Autodesk Inventor part; units mm, degrees
ref_plane "YZ Plane" through (0, 0, 0) normal (1, 0, 0) x (0, 1, 0)
ref_plane "XZ Plane" through (0, 0, 0) normal (0, 1, 0) x (-1, 0, 0)
ref_plane "XY Plane" through (0, 0, 0) normal (0, 0, 1) x (1, 0, 0)
sketch "Schizzo3" plane through (0, 0, 0) normal (0, 0, 1) x (1, 0, 0)
  line L0 (-46, 0) -> (-46, 3)
  line L1 (-46, 3) -> (46, 3)
  line L2 (46, 3) -> (46, 0)
  line L3 (46, 0) -> (61, 0)
  line L4 (61, 0) -> (61, 18)
  line L5 (61, 18) -> (-61, 18)
  line L6 (-61, 18) -> (-61, 0)
  line L7 (-61, 0) -> (-46, 0)
  line L8 (0, 0) -> (0, 18)
  point P0 (0, 3)
  dimension "d10" = 122
  dimension "d11" = 92
  dimension "d12" = 18
  dimension "d13" = 3
extrude "Estrusione1" add sketch "Schizzo3" along normal mid plane 90
sketch "Schizzo4" plane through (-61, 18, 45) normal (0, 1, 0) x (1, 0, 0)
  line L0 (0, 90) -> (0, 0)
  line L1 (0, 90) -> (122, 90)
  line L2 (17, 60) -> (35, 60)
  line L3 (35, 60) -> (35, 30)
  line L4 (35, 30) -> (17, 30)
  line L5 (17, 30) -> (17, 60)
  line L6 (0, 45) -> (122, 45) construction
  line L7 (122, 90) -> (122, 0) construction
  circle A0 centre (17, 60) radius 1.5
  circle A1 centre (35, 60) radius 1.5
  circle A2 centre (35, 30) radius 1.5
  circle A3 centre (17, 30) radius 1.5
  point P0 (61, 45)
  point P1 (26, 68)
  point P2 (44, 80)
  point P3 (44, 68)
  point P4 (102, 80)
  point P5 (102, 68)
  point P6 (18.5, 30)
  point P7 (33.5, 30)
  point P8 (35, 31.5)
  point P9 (35, 58.5)
  point P10 (33.5, 60)
  point P11 (18.5, 60)
  point P12 (17, 58.5)
  point P13 (17, 31.5)
  dimension "d17" = 17
  dimension "d18" = 30
  dimension "d19" = 18
  dimension "d20" = 30
  dimension "d22" = 35
  dimension "d23" = 102
  dimension "d24" = 23
  dimension "d25" = 44
  dimension "d26" = 26
  dimension "d27" = 3
  dimension "d28" = 3
  dimension "d29" = 3
  dimension "d30" = 3
extrude "Estrusione2" cut sketch "Schizzo4" against normal blind 90
hole "Foro1" at (41, 18, -23) at (-17, 18, -23) direction (0, -1, 0) diameter 4.917 end through all
hole "Foro2" at (41, 18, -35) at (-17, 18, -35) direction (0, -1, 0) diameter 4 end through all
pattern_linear "Serie rettangolare1" count 2 spacing 46 along (0, 0, 1) of "Foro1"
pattern_linear "Serie rettangolare2" count 2 spacing 70 along (0, 0, 1) of "Foro2"
sketch "Schizzo5" plane through (-46, 3, 45) normal (0, -1, 0) x (1, 0, 0)
  line L0 (-15, -90) -> (-15, 0)
  line L1 (92, -90) -> (0, -90)
  point P0 (46, -45)
  point P1 (11, -67)
  dimension "d54" = 26
  dimension "d55" = 23
hole "Foro3" at (-35, 3, -22) direction (0, 1, 0) diameter 6.5 end through all counterbore diameter 11 counterbore depth 6.5
pattern_linear "Serie rettangolare3" count 2 spacing 46 along (0, 0, 1) of "Foro3"
properties part number "05-15-2023 esercizi_iogna_serie"
CAD build for the part. Positions are in the model's coordinates, mm. A direction names the side the tool comes from. Round coordinates to 2 decimals unless told otherwise and drop trailing zeros. Order: outer loops, then holes, each group sorted by start corner. A loop starts at its lowest first (then second) coordinate and runs counter-clockwise, first axis right, second up. Notation, with made-up numbers: (30, -37.5) - (76, -37.5) arc R21 cw to (76, -18.5) - close; hole circle Ø5 at (-9.75, 46). An arc over 180 degrees is marked (long way). Answer in a Markdown table with one row per item. Add a question column.
(1) Band-saw the part on C-C on y = 14.75. Count the separate pieces of the cut face and the enclosed holes in it, and give its area (3 significant figures).
(2) Drop a flat-ended pin along its axis: pin 1 Ø3 at (x, z) = (33, -10) entering from -Y. Give the stop position or say it passes through.
(3) 3-axis set-ups, long thin cutter, end or side, ignore diameter. For faces 4 (the face through (-35, 11, 15)), 5 (the face through (46, 2, -1)), 6 (the face through (-40.453, 6.296, 24.716)): which of +Z, -Z, +X, -X, +Y, -Y reach the whole face in a straight line?
(4) Mould opens along X. For faces 1 (the face through (-44, 11, 0)), 2 (the face through (61, 9, -1)), 3 (the face through (-1, 9, 45)) say: +X half, -X half, draft (parallel to the pull), parting line (faces both ways), or undercut.
(5) Probe L1, parallel to Z at x = -17, y = 6; L2, parallel to X at y = 6.5, z = 35; L3, parallel to Z at x = -35, y = 5.5. List the from-to ranges inside material, lowest first. Write a range as [from, to].
(6) Band-saw the part on A-A on x = -35. List the corners of the cut face in (y, z).
(7) Band-saw the part on B-B on z = 35. List the corners of the cut face in (x, y), and give its area (3 significant figures).
(8) Band-saw the part on D-D on z = 0. List the corners of the cut face in (x, y), and give its area (3 significant figures).
Data:
| question | item | result |
|---|---|---|
| 1 | separate pieces | 1 |
| 1 | enclosed holes | 11 |
| 1 | area | 10,200 mm^2 |
| 2 | pin 1 | stops at y = 3 |
| 3 | face 4 | +Y, -Y |
| 3 | face 5 | +Z, -Z, -Y |
| 3 | face 6 | -Y |
| 4 | face 1 | undercut |
| 4 | face 2 | +X half |
| 4 | face 3 | draft |
| 5 | L1 | z = [-45, -37], [-33, -25.46], [-20.54, 20.54], [25.46, 33], [37, 45] |
| 5 | L2 | x = [-61, -19], [-15, 39], [43, 61] |
| 5 | L3 | z = [-45, -27.5], [-16.5, -15], [15, 18.5], [29.5, 45] |
| 6 | outline | (3, -45) - (18, -45) - (18, -25.25) - (9.5, -25.25) - (9.5, -27.5) - (3, -27.5) - close; (3, -16.5) - (9.5, -16.5) - (9.5, -18.75) - (18, -18.75) - (18, -15) - (3, -15) - close; (3, 15) - (18, 15) - (18, 20.75) - (9.5, 20.75) - (9.5, 18.5) - (3, 18.5) - close; (3, 29.5) - (9.5, 29.5) - (9.5, 27.25) - (18, 27.25) - (18, 45) - (3, 45) - close |
| 7 | outline | (-61, 0) - (-46, 0) - (-46, 3) - (-19, 3) - (-19, 18) - (-61, 18) - close; (-15, 3) - (39, 3) - (39, 18) - (-15, 18) - close; (43, 3) - (46, 3) - (46, 0) - (61, 0) - (61, 18) - (43, 18) - close |
| 7 | area | 1,800 mm^2 |
| 8 | outline | (-61, 0) - (-46, 0) - (-46, 3) - (-44, 3) - (-44, 18) - (-61, 18) - close; (-26, 3) - (46, 3) - (46, 0) - (61, 0) - (61, 18) - (-26, 18) - close |
| 8 | area | 1,650 mm^2 |
